Check sheet for the modelled part. Datum: model origin and axes. Units: mm. Face numbers are marked on the shaded views. A direction names the side the tool comes from. Coordinates: 2 decimals unless noted, no trailing zeros. Write each loop counter-clockwise with the first axis right and the second up, starting at its lowest first coordinate (ties: lowest second). Pieces come first, ordered by that corner, then holes. Notation, with made-up numbers: (40.25, -25.5) - (89.25, -25.5) arc R18 ccw to (89.25, -18.5) - close; hole circle Ø4 at (-26.75, 58.5). An arc over 180 degrees is marked (long way). Write each question's results on one line, items separated by ' | '.
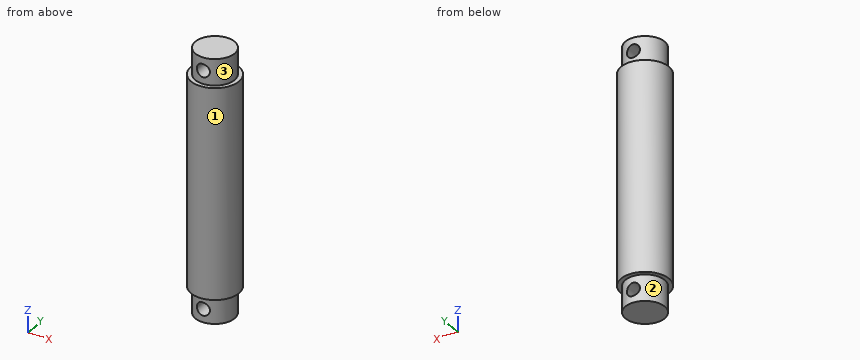
from build123d import *

# Parameters (mm, degrees)
SKETCH1_R               = 5.5
BOSS_EXTRUDE1_DEPTH     = 48
SKETCH2_R               = 4.5
BOSS_EXTRUDE2_DEPTH     = 6
SKETCH3_R               = 4.5
BOSS_EXTRUDE3_DEPTH     = 6
SKETCH4_R               = 1.5
CUT_EXTRUDE1_DEPTH      = 6.5
CUT_EXTRUDE1_DEPTH_BACK = 6.5


with BuildPart() as part:
    # Sketch1 → Boss-Extrude1 (new body)
    with BuildSketch(Plane.XY):
        Circle(SKETCH1_R)
    extrude(amount=BOSS_EXTRUDE1_DEPTH)

    # Sketch2 → Boss-Extrude2 (add)
    with BuildSketch(Plane.XY.offset(48)):
        Circle(SKETCH2_R)
    extrude(amount=BOSS_EXTRUDE2_DEPTH)

    # Sketch3 → Boss-Extrude3 (add)
    with BuildSketch(Plane(origin=(0, 0, 0), x_dir=(-1, 0, 0), z_dir=(0, 0, -1))):
        Circle(SKETCH3_R)
    extrude(amount=BOSS_EXTRUDE3_DEPTH)

    # Sketch4 → Cut-Extrude1 (cut, two sides)
    with BuildSketch(Plane(origin=(0, 0, 0), x_dir=(1, 0, 0), z_dir=(0, 1, 0))) as cut_extrude1_sk:
        with Locations((0, 3)):
            Circle(SKETCH4_R)
        with Locations((0, -51)):
            Circle(SKETCH4_R)
    extrude(amount=CUT_EXTRUDE1_DEPTH, mode=Mode.SUBTRACT)
    extrude(cut_extrude1_sk.sketch, amount=-CUT_EXTRUDE1_DEPTH_BACK, mode=Mode.SUBTRACT)


solid = part.part
1. Sectioned sample at C-C (z = 51). Record the cut outline in (x, y), then the cut area to 3 significant figures.
Values follow:
outline: (-1.5, -4.24) - (-1.5, 4.24) arc R4.5 ccw to start; (1.5, -4.24) arc R4.5 ccw to (1.5, 4.24) - close | area: 37.1 mm^2
2. Access from +Z, -Z, +X, -X, +Y, -Y to the whole of each face (thin tool, end or side, straight path). Record for the marked faces 1, 2 and 3.
Values follow:
face 1: +Z, -Z | face 2: -Z | face 3: +Z
3. Go/stop test with flat-tipped pins: pin 1 (2 mm diameter, centred on y = -3, z = 47.5, fed in from +X); pin 2 (5 mm diameter, centred on x = 0, z = -3, fed in from -Y); pin 3 (1 mm diameter, centred on y = 3.5, z = 20.5, fed in from -X). Record where each tip stops, or that it passes through.
Values follow:
pin 1: stops at x = 5.12 | pin 2: stops at y = -4.5 | pin 3: stops at x = -4.61
4. Sectioned sample at A-A (y = 0). Record the cut outline in (x, z), then the cut area to 3 significant figures.
Values follow:
outline: (-5.5, 0) - (-4.5, 0) - (-4.5, -6) - (4.5, -6) - (4.5, 0) - (5.5, 0) - (5.5, 48) - (4.5, 48) - (4.5, 54) - (-4.5, 54) - (-4.5, 48) - (-5.5, 48) - close; hole circle Ø3 at (0, -3); hole circle Ø3 at (0, 51) | area: 622 mm^2
5. Material ranges on L1, parallel to Z at x = 0, y = -2.5; L2, parallel to Z at x = -1.25, y = 3.75; L3, parallel to X at y = -1.5, z = 51, recorded low to high. Write a range as [from, to].
Values follow:
L1: z = [-6, -4.5], [-1.5, 49.5], [52.5, 54] | L2: z = [-6, -3.83], [-2.17, 50.17], [51.83, 54] | L3: x = [-4.24, -1.5], [1.5, 4.24]
6. Sectioned sample at D-D (x = 2.25). Record the cut outline in (y, z).
Values follow:
outline: (-5.02, 0) - (-3.9, 0) - (-3.9, -6) - (3.9, -6) - (3.9, 0) - (5.02, 0) - (5.02, 48) - (3.9, 48) - (3.9, 54) - (-3.9, 54) - (-3.9, 48) - (-5.02, 48) - close
7. Sectioned sample at B-B (x = 0). Record the cut outline in (y, z), then the cut area to 3 significant figures.
Values follow:
outline: (-5.5, 0) - (-4.5, 0) - (-4.5, -1.5) - (4.5, -1.5) - (4.5, 0) - (5.5, 0) - (5.5, 48) - (4.5, 48) - (4.5, 49.5) - (-4.5, 49.5) - (-4.5, 48) - (-5.5, 48) - close; (-4.5, -6) - (4.5, -6) - (4.5, -4.5) - (-4.5, -4.5) - close; (-4.5, 52.5) - (4.5, 52.5) - (4.5, 54) - (-4.5, 54) - close | area: 582 mm^2
